from build123d import *

# Parameters (mm, degrees)
F0_W        = 201.6125
F0_H        = 482.6
F1_DEPTH    = 0.79375
F3_DEPTH    = 201.6125
F4_T1_DEPTH = 508.79375
F4_T3_DEPTH = 508.79375
F5_R        = 2.15265
F6_DEPTH    = 0.79375


# Not quite as in the source:
# - a fillet or chamfer that OpenCascade refuses, or shapes differently, is made with other operations: its cross-section is extruded or revolved along the edge and cut away or added


with BuildPart() as f1:
    # F0 (on Top) → F1 (new body)
    with BuildSketch(Plane.XY):
        Rectangle(F0_W, F0_H)
    extrude(amount=F1_DEPTH)

    # F2 (on face) → F3 (join, through all)
    with BuildSketch(Plane.YZ.offset(100.80625)):
        with BuildLine():
            ThreePointArc((244.0671948322, 0.9145683356), (242.6849155488, 0.8239689648), (241.3, 0.79375))
            Line((241.3, 0.79375), (241.3, 0))
            ThreePointArc((241.3, 0), (242.7195384376, 0.0309744389), (244.136374703, 0.123838794))
            Line((244.136374703, 0.123838794), (294.7430653661, 4.5513505256))
            ThreePointArc((294.7430653661, 4.5513505256), (298.5031396949, 4.5918955138), (302.2254864388, 4.0590375853))
            Line((302.2254864388, 4.0590375853), (413.8036674178, -20.7361137434))
            Line((413.8036674178, -20.7361137434), (413.9758559687, -19.9612652644))
            Line((413.9758559687, -19.9612652644), (302.3976749897, 4.8338860643))
            ThreePointArc((302.3976749897, 4.8338860643), (298.5552525443, 5.3839329582), (294.6738854953, 5.3420800672))
            Line((294.6738854953, 5.3420800672), (244.0671948322, 0.9145683356))
        make_face()
        with BuildLine():
            Line((-241.3, 0), (-241.3, 0.79375))
            ThreePointArc((-241.3, 0.79375), (-242.6849155488, 0.8239689648), (-244.0671948322, 0.9145683356))
            Line((-244.0671948322, 0.9145683356), (-294.6738854953, 5.3420800672))
            ThreePointArc((-294.6738854953, 5.3420800672), (-299.6272962644, 5.3969871417), (-304.5316552149, 4.699451251))
            Line((-304.5316552149, 4.699451251), (-416.1396714134, -19.9610580753))
            Line((-416.1396714134, -19.9610580753), (-415.9684178764, -20.7361137434))
            Line((-415.9684178764, -20.7361137434), (-304.3604016779, 3.924395583))
            ThreePointArc((-304.3604016779, 3.924395583), (-299.5756612384, 4.6049184032), (-294.7430653661, 4.5513505256))
            Line((-294.7430653661, 4.5513505256), (-244.136374703, 0.123838794))
            ThreePointArc((-244.136374703, 0.123838794), (-242.7195384376, 0.0309744389), (-241.3, 0))
        make_face()
    extrude(amount=-F3_DEPTH)

    # F4: fillet of radius 101.6 on 4 edges, made by hand

    # F4_s2 → F4_t1 (cut)
    with BuildSketch(Plane(origin=(0, -40.0183995531, -180.082797989), x_dir=(1, 0, 0), z_dir=(0, 0.2169304578, 0.9761870602))):
        with BuildLine():
            ThreePointArc((100.80625, 306.8480802377), (71.0482989686, 378.6901292062), (-0.79375, 408.4480802377))
            Line((-0.79375, 408.4480802377), (100.80625, 408.4480802377))
            Line((100.80625, 408.4480802377), (100.80625, 306.8480802377))
        make_face()
        with BuildLine():
            ThreePointArc((0.79375, 408.4480802377), (-71.0482989686, 378.6901292062), (-100.80625, 306.8480802377))
            Line((-100.80625, 306.8480802377), (-100.80625, 408.4480802377))
            Line((-100.80625, 408.4480802377), (0.79375, 408.4480802377))
        make_face()
    extrude(amount=F4_T1_DEPTH, mode=Mode.SUBTRACT)

    # F4_s4 → F4_t3 (cut)
    with BuildSketch(Plane(origin=(0, -69.9668558158, 316.6545294712), x_dir=(1, 0, 0), z_dir=(0, 0.2157524875, -0.9764480857))):
        with BuildLine():
            ThreePointArc((100.80625, 309.0454334801), (71.0482989686, 380.8874824486), (-0.79375, 410.6454334801))
            Line((-0.79375, 410.6454334801), (100.80625, 410.6454334801))
            Line((100.80625, 410.6454334801), (100.80625, 309.0454334801))
        make_face()
        with BuildLine():
            ThreePointArc((0.79375, 410.6454334801), (-71.0482989686, 380.8874824486), (-100.80625, 309.0454334801))
            Line((-100.80625, 309.0454334801), (-100.80625, 410.6454334801))
            Line((-100.80625, 410.6454334801), (0.79375, 410.6454334801))
        make_face()
    extrude(amount=F4_T3_DEPTH, mode=Mode.SUBTRACT)

    # F5 (on face) → F6 (cut, through all)
    with BuildSketch(Plane.XY.offset(0.79375)):
        with Locations((-11.1125, 237.33125)):
            Circle(F5_R)
        with Locations((11.1125, 237.33125)):
            Circle(F5_R)
        with Locations((11.1125, 223.04375)):
            Circle(F5_R)
        with Locations((-11.1125, 223.04375)):
            Circle(F5_R)
        with Locations((11.1125, -223.04375)):
            Circle(F5_R)
        with Locations((-11.1125, -223.04375)):
            Circle(F5_R)
        with Locations((-11.1125, -237.33125)):
            Circle(F5_R)
        with Locations((11.1125, -237.33125)):
            Circle(F5_R)
    extrude(amount=-F6_DEPTH, mode=Mode.SUBTRACT)


solid = f1.part
Source: CAD feature listing. Evaluate the final solid. Frame: model axes, mm. A direction names the side the tool comes from. Coordinates: 2 decimals unless noted, no trailing zeros. Loops run counter-clockwise (first coordinate to the right, second up) from the corner with the lowest first, then second, coordinate; pieces in that order, holes last. Notation, with made-up numbers: (-29, -39) -> (-17, -39) arc R23 cw to (-17, -17) -> close; hole circle Ø9 at (11, 33.5). An arc over 180 degrees is marked (long way). Answer in a Markdown table with one row per item. Add a question column.
Q1. Section A-A on x = 89.5. Return the cut outline in (y, z), and give its area (3 significant figures).
Q2. Contact query for flat-ended pins moving along their axis: pin 1 Ø6 at (y, z) = (239, -3.5) entering from +X; pin 2 Ø5 at (x, y) = (-11.11, 223.04) entering from -Z; pin 3 Ø5.5 at (x, y) = (-11.11, -237.33) entering from +Z. Output: stop coordinate, or through.
Q3. Ray query, line 1 along Z through (x, y) = (85.5, 320); line 2 along Z through (x, y) = (-5, 156). Return the intervals inside material, ascending.
Q4. Section B-B on y = -180.5. Return the cut outline in (x, z).
Q5. Reachability of faces 1 (the face through (72.107, 383.79, -13.666)), 2 (the face through (-1, 3, 0.794)), 3 (the face through (1.41, -269.79, 2.37)) from +Z, -Z, +X, -X, +Y, -Y: full face, straight path, thin tool, end or side. Return the list, or none.
Q6. Pull-direction query (Y, two-part tool) for faces 4 (the face through (72.107, -385.949, -13.691)), 5 (the face through (1.411, -348.544, -5.838)), 6 (the face through (1.411, 346.569, -4.982)); classes: pulls with the +Y half, pulls with the -Y half, needs draft (parallel to the pull), parting line crosses it, or undercut.
Q7. Section C-C on x = -27.5. Return the cut outline in (y, z).
Computed values:
| question | item | result |
|---|---|---|
| 1 | outline | (-362.41, -8.09) -> (-362.24, -8.87) -> (-304.36, 3.92) arc R31.75 cw to (-294.74, 4.55) -> (-244.14, 0.12) arc R32.54 ccw to (-241.3, 0) -> (241.3, 0) arc R32.54 ccw to (244.14, 0.12) -> (294.74, 4.55) arc R24.61 cw to (302.23, 4.06) -> (360.09, -8.8) -> (360.27, -8.03) -> (302.4, 4.83) arc R25.4 ccw to (294.67, 5.34) -> (244.07, 0.91) arc R31.75 cw to (241.3, 0.79) -> (-241.3, 0.79) arc R31.75 cw to (-244.07, 0.91) -> (-294.67, 5.34) arc R32.54 ccw to (-304.53, 4.7) -> close |
| 1 | area | 576 mm^2 |
| 2 | pin 1 | passes through |
| 2 | pin 2 | stops at z = 0 |
| 2 | pin 3 | stops at z = 0.79 |
| 3 | line 1 | z = 0.11 to 0.92 |
| 3 | line 2 | z = 0 to 0.79 |
| 4 | outline | (-100.81, 0) -> (100.81, 0) -> (100.81, 0.79) -> (-100.81, 0.79) -> close |
| 5 | face 1 | -Z, +X, +Y |
| 5 | face 2 | +Z, +X, -X |
| 5 | face 3 | -Z, +X, -X |
| 6 | face 4 | pulls with the -Y half |
| 6 | face 5 | undercut |
| 6 | face 6 | pulls with the +Y half |
| 7 | outline | (-412.22, -19.09) -> (-412.04, -19.87) -> (-304.36, 3.92) arc R31.75 cw to (-294.74, 4.55) -> (-244.14, 0.12) arc R32.54 ccw to (-241.3, 0) -> (241.3, 0) arc R32.54 ccw to (244.14, 0.12) -> (294.74, 4.55) arc R24.61 cw to (302.23, 4.06) -> (409.88, -19.86) -> (410.05, -19.09) -> (302.4, 4.83) arc R25.4 ccw to (294.67, 5.34) -> (244.07, 0.91) arc R31.75 cw to (241.3, 0.79) -> (-241.3, 0.79) arc R31.75 cw to (-244.07, 0.91) -> (-294.67, 5.34) arc R32.54 ccw to (-304.53, 4.7) -> close |
